```python
from build123d import *
from build123d.topology import SkipClean

# Parameters (mm, degrees)
SKETCH1_W                 = 31
SKETCH1_H                 = 22
BOSS_EXTRUDE1_DEPTH       = 11
SKETCH2_W                 = 31
SKETCH2_H                 = 22
SKETCH2_R                 = 7.843750423
BOSS_EXTRUDE2_DEPTH       = 5
SKETCH3_W                 = 24.5
SKETCH3_H                 = 15.5
CUT_EXTRUDE1_DEPTH        = 7.75
FILLET1_R                 = 7.75
CUT_EXTRUDE2_DEPTH        = 32.812929761
CUT_EXTRUDE2_DEPTH_BACK   = 32.812929761
SKETCH4_R                 = 5
SKETCH5_W                 = 8
SKETCH5_H                 = 8
SKETCH5_R                 = 1.905800151
BOSS_EXTRUDE3_DEPTH       = 6
CUT_EXTRUDE3_START        = -3
SKETCH6_R                 = 3
SKETCH6_R_2               = 1.905800151
CUT_EXTRUDE3_DEPTH        = 3
MIRROR9_COPY_1_SKETCH_W   = 8
MIRROR9_COPY_1_SKETCH_H   = 8
MIRROR9_COPY_1_SKETCH_R   = 1.905800151
MIRROR9_COPY_1_DEPTH      = 6
MIRROR9_START             = -3
MIRROR9_COPY_2_SKETCH_R   = 3
MIRROR9_COPY_2_SKETCH_R_2 = 1.905800151
MIRROR9_COPY_2_DEPTH      = 3
CHAMFER2_SIZE             = 4
SKETCH8_R                 = 3
BOSS_EXTRUDE4_DEPTH       = 16
SKETCH9_R                 = 1.75
BOSS_EXTRUDE5_DEPTH       = 16
CUT_EXTRUDE6_DEPTH        = 9
SKETCH11_R                = 1.75
CUT_EXTRUDE7_DEPTH        = 8
FILLET2_R                 = 2
CUT_EXTRUDE8_DEPTH        = 41.425858061
CUT_EXTRUDE8_DEPTH_BACK   = 41.425858061
SKETCH12_R                = 1.75
CUT_EXTRUDE9_START        = -3
SKETCH13_R                = 1.75
CUT_EXTRUDE9_DEPTH        = 3
BOSS_EXTRUDE8_DEPTH       = 4
BOSS_EXTRUDE9_DEPTH       = 4
CUT_EXTRUDE11_START       = -5
SKETCH18_R                = 1.75
CUT_EXTRUDE11_DEPTH       = 5
SKETCH20_W                = 15
SKETCH20_H                = 2
CUT_EXTRUDE12_DEPTH       = 12


with BuildPart() as part:
    # Sketch1 → Boss-Extrude1 (new body)
    with BuildSketch(Plane(origin=(0, 0, 0), x_dir=(1, 0, 0), z_dir=(0, 1, 0))):
        Rectangle(SKETCH1_W, SKETCH1_H)
    extrude(amount=BOSS_EXTRUDE1_DEPTH)

    # Sketch2 → Boss-Extrude2 (add)
    with BuildSketch(Plane(origin=(0, 0, 0), x_dir=(1, 0, 0), z_dir=(0, 1, 0))):
        Rectangle(SKETCH2_W, SKETCH2_H)
        with Locations(Location((0, 0, 0), (0, 0, 270))):
            Circle(SKETCH2_R, mode=Mode.SUBTRACT)
    extrude(amount=-BOSS_EXTRUDE2_DEPTH)

    # Sketch3 → Cut-Extrude1 (cut)
    with BuildSketch(Plane(origin=(0, 11, 0), x_dir=(1, 0, 0), z_dir=(0, 1, 0))):
        Rectangle(SKETCH3_W, SKETCH3_H)
    extrude(amount=-CUT_EXTRUDE1_DEPTH, mode=Mode.SUBTRACT)

    # Fillet1
    fillet1_edges = [part.edges().sort_by_distance(p)[0] for p in [
        (0, 3.25, 7.75),
        (0, 3.25, -7.75),
    ]]
    fillet(fillet1_edges, radius=FILLET1_R - 0.0001)  # a hair under: the kernel refuses the full size

    # Sketch4 → Cut-Extrude2 (cut, two sides: drawn at the far end of the back side and taken through both)
    with BuildSketch(Plane(origin=(-12.25, 0, 0), x_dir=(0, 0, -1), z_dir=(1, 0, 0)).offset(-CUT_EXTRUDE2_DEPTH_BACK)):
        with Locations((0, 11)):
            Circle(SKETCH4_R)
    extrude(amount=CUT_EXTRUDE2_DEPTH + CUT_EXTRUDE2_DEPTH_BACK, mode=Mode.SUBTRACT)

    # Sketch5 → Boss-Extrude3 (add)
    with BuildSketch(Plane(origin=(0, 11, 0), x_dir=(1, 0, 0), z_dir=(0, 1, 0))):
        with Locations((11.5, -15)):
            Rectangle(SKETCH5_W, SKETCH5_H)
        with Locations(Location((11.5, -15, 0), (0, 0, 270))):
            Circle(SKETCH5_R, mode=Mode.SUBTRACT)
    boss_extrude3 = extrude(amount=-BOSS_EXTRUDE3_DEPTH)

    # Sketch6 → Cut-Extrude3 (cut)
    with BuildSketch(Plane.XZ.offset(-5).offset(CUT_EXTRUDE3_START)):
        with Locations(Location((11.5, 15, 0), (0, 0, 270))):
            Circle(SKETCH6_R)
        with Locations(Location((11.5, 15, 0), (0, 0, 90))):
            Circle(SKETCH6_R_2, mode=Mode.SUBTRACT)
    cut_extrude3 = extrude(amount=CUT_EXTRUDE3_DEPTH, mode=Mode.SUBTRACT)

    # Mirror8: Boss-Extrude3, Cut-Extrude3 across plane
    add(boss_extrude3.mirror(Plane(origin=(0, 0, 0), x_dir=(0, 0, 1), z_dir=(1, 0, 0))))
    add(cut_extrude3.mirror(Plane(origin=(0, 0, 0), x_dir=(0, 0, 1), z_dir=(1, 0, 0))), mode=Mode.SUBTRACT)

    # Mirror9: Boss-Extrude3, Cut-Extrude3 across plane
    add(boss_extrude3.mirror(Plane.XY))
    add(cut_extrude3.mirror(Plane.XY), mode=Mode.SUBTRACT)

    # Mirror9 copy 1 sketch → Mirror9 copy 1 (add)
    with BuildSketch(Plane(origin=(0, 11, 0), x_dir=(-1, 0, 0), z_dir=(0, 1, 0))):
        with Locations((11.5, -15)):
            Rectangle(MIRROR9_COPY_1_SKETCH_W, MIRROR9_COPY_1_SKETCH_H)
        with Locations(Location((11.5, -15, 0), (0, 0, 270))):
            Circle(MIRROR9_COPY_1_SKETCH_R, mode=Mode.SUBTRACT)
    extrude(amount=-MIRROR9_COPY_1_DEPTH)

    # Mirror9 copy 2 sketch → Mirror9 copy 2 (cut)
    with BuildSketch(Plane(origin=(0, 5, 0), x_dir=(-1, 0, 0), z_dir=(0, -1, 0)).offset(MIRROR9_START)):
        with Locations(Location((11.5, 15, 0), (0, 0, 270))):
            Circle(MIRROR9_COPY_2_SKETCH_R)
        with Locations(Location((11.5, 15, 0), (0, 0, 90))):
            Circle(MIRROR9_COPY_2_SKETCH_R_2, mode=Mode.SUBTRACT)
    extrude(amount=MIRROR9_COPY_2_DEPTH, mode=Mode.SUBTRACT)

    # Chamfer2
    chamfer2_edges = [part.edges().sort_by_distance(p)[0] for p in [
        (-7.5, 8, -11),
        (7.5, 8, -11),
        (7.5, 8, 11),
        (-7.5, 8, 11),
    ]]
    chamfer(chamfer2_edges, length=CHAMFER2_SIZE)

    # Sketch8 → Boss-Extrude4 (add)
    # profile 1 of 3: a face of its own
    with BuildSketch(Plane(origin=(0, 11, 0), x_dir=(1, 0, 0), z_dir=(0, 1, 0))):
        Polygon((3.5, -11), (-3.5, -11), (-7.5, -15), (-7.5, -19), (7.5, -19), (7.5, -15), align=None)
    # profile 2 of 3: a face of its own
    with BuildSketch(Plane(origin=(0, 11, 0), x_dir=(1, 0, 0), z_dir=(0, 1, 0))):
        Polygon((15.5, -11), (3.5, -11), (7.5, -15), (7.5, -19), (15.5, -19), align=None)
        with Locations(Location((11.5, -15, 0), (0, 0, 90))):
            Circle(SKETCH8_R, mode=Mode.SUBTRACT)
    # profile 3 of 3: a face of its own
    with BuildSketch(Plane(origin=(0, 11, 0), x_dir=(1, 0, 0), z_dir=(0, 1, 0))):
        Polygon((-3.5, -11), (-15.5, -11), (-15.5, -19), (-7.5, -19), (-7.5, -15), align=None)
        with Locations(Location((-11.5, -15, 0), (0, 0, 90))):
            Circle(SKETCH8_R, mode=Mode.SUBTRACT)
    extrude(amount=-BOSS_EXTRUDE4_DEPTH)

    # Sketch9 → Boss-Extrude5 (add)
    with BuildSketch(Plane.ZY.offset(15.5)):
        Polygon((19, 11), (19, 1), (35, 1), (35, 17), (19, 17), align=None)
        with Locations((29, 9)):
            Circle(SKETCH9_R, mode=Mode.SUBTRACT)
    extrude(amount=-BOSS_EXTRUDE5_DEPTH)

    # Sketch10 → Cut-Extrude6 (cut)
    with BuildSketch(Plane(origin=(0, 17, 0), x_dir=(1, 0, 0), z_dir=(0, 1, 0))):
        with BuildLine():
            ThreePointArc((-11.227178029, -24.25), (-11.5, -23), (-11.227178029, -21.75))
            Line((-11.227178029, -21.75), (-15.5, -21.75))
            Line((-15.5, -21.75), (-15.5, -24.25))
            Line((-15.5, -24.25), (-11.227178029, -24.25))
        make_face()
        with BuildLine():
            Line((-8.5, -24.25), (-8.5, -21.75))
            Line((-8.5, -21.75), (-11.227178029, -21.75))
            ThreePointArc((-11.227178029, -21.75), (-11.5, -23), (-11.227178029, -24.25))
            Line((-11.227178029, -24.25), (-8.5, -24.25))
        make_face()
        with BuildLine():
            Line((-11.227178029, -21.75), (-8.5, -21.75))
            Line((-8.5, -21.75), (-8.5, -24.25))
            Line((-8.5, -24.25), (-11.227178029, -24.25))
            ThreePointArc((-11.227178029, -24.25), (-7.860286817, -25.931001031), (-5.5, -23))
            ThreePointArc((-5.5, -23), (-7.860286817, -20.068998969), (-11.227178029, -21.75))
        make_face()
    extrude(amount=-CUT_EXTRUDE6_DEPTH, mode=Mode.SUBTRACT)

    # Sketch11 → Cut-Extrude7 (cut)
    with BuildSketch(Plane.ZY.offset(15.5)):
        Polygon((29, 12.175426481), (26.25, 10.58771324), (26.25, 7.41228676), (29, 5.824573519), (31.75, 7.41228676), (31.75, 10.58771324), align=None)
        with Locations((29, 9)):
            Circle(SKETCH11_R, mode=Mode.SUBTRACT)
    extrude(amount=-CUT_EXTRUDE7_DEPTH, mode=Mode.SUBTRACT)

    # Fillet2
    fillet2_edges = [part.edges().sort_by_distance(p)[0] for p in [
        (-11.227178029, 12.5, 21.75),
        (-11.227178029, 12.5, 24.25),
    ]]
    fillet(fillet2_edges, radius=FILLET2_R)

    # Sketch12 → Cut-Extrude8 (cut, two sides: drawn at the far end of the back side and taken through both)
    with BuildSketch(Plane(origin=(0, 8, 0), x_dir=(1, 0, 0), z_dir=(0, 1, 0)).offset(-CUT_EXTRUDE8_DEPTH_BACK)):
        with Locations(Location((-8.5, -23, 0), (0, 0, 90))):
            Circle(SKETCH12_R)
    extrude(amount=CUT_EXTRUDE8_DEPTH + CUT_EXTRUDE8_DEPTH_BACK, mode=Mode.SUBTRACT)

    # Sketch13 → Cut-Extrude9 (cut)
    with BuildSketch(Plane.XZ.offset(-1).offset(CUT_EXTRUDE9_START)):
        Polygon((-5.324573519, 23), (-6.91228676, 25.75), (-10.08771324, 25.75), (-11.675426481, 23), (-10.08771324, 20.25), (-6.91228676, 20.25), align=None)
        with Locations(Location((-8.5, 23, 0), (0, 0, 270))):
            Circle(SKETCH13_R, mode=Mode.SUBTRACT)
    extrude(amount=CUT_EXTRUDE9_DEPTH, mode=Mode.SUBTRACT)

    # Sketch15 → Boss-Extrude8 (add)
    with SkipClean():  # the faces are left unmerged after this step: merging them gives an invalid solid
        with BuildSketch(Plane.ZY.offset(15.5)):
            with BuildLine():
                Line((24.25, 17), (24.25, 8))
                Line((24.25, 8), (21.75, 8))
                Line((21.75, 8), (21.75, 17))
                Line((21.75, 17), (19, 17))
                Line((19, 17), (19, 11))
                Line((19, 11), (5, 11))
                ThreePointArc((5, 11), (0, 6), (-5, 11))
                Line((-5, 11), (-19, 11))
                Line((-19, 11), (-19, 5))
                Line((-19, 5), (-11, 5))
                Line((-11, 5), (-11, -5))
                Line((-11, -5), (19, -5))
                Line((19, -5), (19, 1))
                Line((19, 1), (35, 1))
                Line((35, 1), (35, 17))
                Line((35, 17), (24.25, 17))
            make_face()
            Polygon((29, 12.175426481), (26.25, 10.58771324), (26.25, 7.41228676), (29, 5.824573519), (31.75, 7.41228676), (31.75, 10.58771324), align=None, mode=Mode.SUBTRACT)
        extrude(amount=BOSS_EXTRUDE8_DEPTH)
    add(part.part.scale(1), mode=Mode.REPLACE)  # the faces are merged on a copy

    # Sketch17 → Boss-Extrude9 (add)
    with BuildSketch(Plane(origin=(15.5, 0, 0), x_dir=(0, 0, -1), z_dir=(1, 0, 0))):
        with BuildLine():
            Line((-5, 11), (-19, 11))
            Line((-19, 11), (-19, -5))
            Line((-19, -5), (11, -5))
            Line((11, -5), (11, 5))
            Line((11, 5), (19, 5))
            Line((19, 5), (19, 11))
            Line((19, 11), (5, 11))
            ThreePointArc((5, 11), (0, 6), (-5, 11))
        make_face()
    extrude(amount=BOSS_EXTRUDE9_DEPTH)

    # Sketch18 → Cut-Extrude11 (cut)
    with BuildSketch(Plane(origin=(0.5, 0, 0), x_dir=(0, 0, -1), z_dir=(1, 0, 0)).offset(CUT_EXTRUDE11_START)):
        Polygon((-35, 1), (-19, 1), (-19, 11), (-19, 17), (-35, 17), align=None)
        with Locations(Location((-29, 9, 0), (0, 0, 180))):
            Circle(SKETCH18_R, mode=Mode.SUBTRACT)
    extrude(amount=CUT_EXTRUDE11_DEPTH, mode=Mode.SUBTRACT)

    # Sketch20 → Cut-Extrude12 (cut)
    with BuildSketch(Plane(origin=(0, 17, 0), x_dir=(1, 0, 0), z_dir=(0, 1, 0))):
        with Locations((-12, -34)):
            Rectangle(SKETCH20_W, SKETCH20_H)
    extrude(amount=-CUT_EXTRUDE12_DEPTH, mode=Mode.SUBTRACT)


solid = part.part
```
Check sheet for the modelled part. Datum: model origin and axes. Units: mm. A direction names the side the tool comes from. Round coordinates to 2 decimals unless told otherwise and drop trailing zeros. Order: outer loops, then holes, each group sorted by start corner. A loop starts at its lowest first (then second) coordinate and runs counter-clockwise, first axis right, second up.
1) Tool access check on faces 1 (the flat face through (-7.1, 4, 24.3)), 2 (the cylindrical face through (0.17, 5.58, -5.54)), 3 (the flat face through (0, 11, 12)), 4 (the flat face through (-5.5, 8, -13)), 5 (the flat face through (-12, 1, 27)). Record the directions out of +Z, -Z, +X, -X, +Y, -Y that give a thin tool (end or side, any length) a straight path to the whole face; none if there is none.
2) Section check B-B (z = 15). Record the boundary of the cut face in (x, y), and give its area (3 significant figures).
3) Section check C-C (x = 15.5). Record the boundary of the cut face in (y, z), and give its area (3 significant figures).
4) Mould release check, pull along Z, two halves, no side actions. Record for faces 6 (the flat face through (-12, 14, 19)), 7 (the flat face through (-12, 11, 33)), 8 (the flat face through (0, 0, 0)): +Z half, -Z half, draft (parallel to the pull), parting line (faces both ways), or undercut.
5) Go/stop test with flat-tipped pins: pin 1 Ø7 at (x, z) = (5.5, 11.5) entering from +Y; pin 2 Ø12 at (x, y) = (10, 12.5) entering from -Z; pin 3 Ø12.5 at (x, z) = (0, 0) entering from +Y; pin 4 Ø1.6 at (x, y) = (-12, 9.5) entering from +Z. Record where each tip stops, or that it passes through.
6) Section check A-A (x = 11.5). Give the number of separate pieces and of enclosed holes in the cut face, and give its area (3 significant figures).
7) Scan lines: line 1 (X direction, y = 6.25, z = -2); line 2 (X direction, y = 10.3, z = 15); line 3 (X direction, y = 6.45, z = 23). Record each from-to range of solid material in increasing order.
Result:
1. face 1: -Y
1. face 2: +Y
1. face 3: -Z, +X, -X, +Y
1. face 4: -Z, +Y, -Y
1. face 5: +Z, +X, -X, -Y
2. outline: (-19.5, -5) - (-14.5, -5) - (-14.5, 8) - (-13.41, 8) - (-13.41, 11) - (-19.5, 11) - close; (-9.59, 8) - (-8.5, 8) - (-8.5, -5) - (8.5, -5) - (8.5, 8) - (9.59, 8) - (9.59, 11) - (-9.59, 11) - close; (13.41, 8) - (14.5, 8) - (14.5, -5) - (19.5, -5) - (19.5, 11) - (13.41, 11) - close
2. area: 445 mm2
3. outline: (-5, -11) - (5, -11) - (5, -19) - (11, -19) - (11, -5) arc R5 cw to (11, 5) - (11, 19) - (-5, 19) - close
3. area: 489 mm2
4. face 6: -Z half
4. face 7: +Z half
4. face 8: undercut
5. pin 1: stops at y = 11
5. pin 2: stops at z = -19
5. pin 3: stops at y = 6.42
5. pin 4: stops at z = 33
6. separate pieces: 3
6. enclosed holes: 0
6. area: 315 mm2
7. line 1: x = -19.5 to -12.25, 12.25 to 19.5
7. line 2: x = -19.5 to -13.41, -9.59 to 9.59, 13.41 to 19.5
7. line 3: x = -19.5 to -10.25, -6.75 to -4.5
